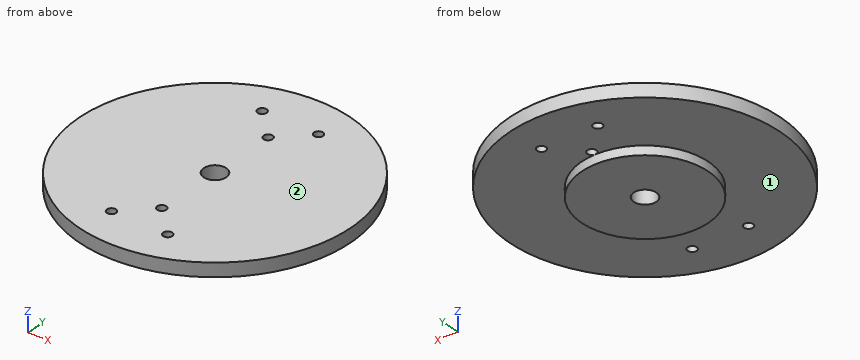
```python
from build123d import *

# Parameters (mm, degrees)
SKETCH1_R                = 76.2
SKETCH1_R_2              = 38.1
SKETCH1_R_3              = 12.7
SKETCH1_R_4              = 6.35
BOSS_EXTRUDE1_DEPTH      = 7.62
SKETCH2_R                = 35.56
BOSS_EXTRUDE2_DEPTH      = 5.08
CUT_EXTRUDE2_START       = -12.7
CUT_EXTRUDE2_OUTLINE_R   = 6.35
CUT_EXTRUDE2_OUTLINE_R_2 = 2.54
CUT_EXTRUDE2_DEPTH       = 12.7


# Read off the part's stored shape, not the designer's step: Cut-Extrude2
with BuildPart() as part:
    # Sketch1 → Boss-Extrude1 (new body)
    # profile 1 of 3: a face of its own
    with BuildSketch(Plane.XY):
        with Locations(Location((0, 0, 0), (0, 0, 180))):
            Circle(SKETCH1_R)
        Circle(SKETCH1_R_2, mode=Mode.SUBTRACT)
    # profile 2 of 3: a face of its own
    with BuildSketch(Plane.XY):
        Circle(SKETCH1_R_2)
        Circle(SKETCH1_R_3, mode=Mode.SUBTRACT)
    # profile 3 of 3: a face of its own
    with BuildSketch(Plane.XY):
        Circle(SKETCH1_R_3)
        with Locations(Location((0, 0, 0), (0, 0, 180))):
            Circle(SKETCH1_R_4, mode=Mode.SUBTRACT)
    extrude(amount=BOSS_EXTRUDE1_DEPTH)

    # Sketch2 → Boss-Extrude2 (add)
    with BuildSketch(Plane(origin=(0, 0, 0), x_dir=(-1, 0, 0), z_dir=(0, 0, -1))):
        with Locations(Location((0, 0, 0), (0, 0, 180))):
            Circle(SKETCH2_R)
    extrude(amount=BOSS_EXTRUDE2_DEPTH)

    # Cut-Extrude2 outline → Cut-Extrude2 (cut)
    with BuildSketch(Plane.XY.offset(7.62).offset(CUT_EXTRUDE2_START)):
        Circle(CUT_EXTRUDE2_OUTLINE_R)
        with Locations((-15.875, -53.975)):
            Circle(CUT_EXTRUDE2_OUTLINE_R_2)
        with Locations((0, -38.1)):
            Circle(CUT_EXTRUDE2_OUTLINE_R_2)
        with Locations((-15.875, 53.975)):
            Circle(CUT_EXTRUDE2_OUTLINE_R_2)
        with Locations((0, 38.1)):
            Circle(CUT_EXTRUDE2_OUTLINE_R_2)
        with Locations((15.875, 53.975)):
            Circle(CUT_EXTRUDE2_OUTLINE_R_2)
        with Locations((15.875, -53.975)):
            Circle(CUT_EXTRUDE2_OUTLINE_R_2)
    extrude(amount=CUT_EXTRUDE2_DEPTH, mode=Mode.SUBTRACT)


solid = part.part
```
CAD build for the part. Positions are in the model's coordinates, mm. Face numbers are marked on the shaded views. A direction names the side the tool comes from. Round coordinates to 2 decimals unless told otherwise and drop trailing zeros. Loops run counter-clockwise (first coordinate to the right, second up) from the corner with the lowest first, then second, coordinate; pieces in that order, holes last. Notation, with made-up numbers: M 71.5,-37.75 L 116.5,-37.75 A19 ccw 116.5,-33.75 Z; hole C 81,5.5 d10. An arc over 180 degrees is marked long. Use a Markdown table: item, result. Add a question column.
(1) Cut at A-A (y = 0). Give the cut face in (x, z).
(2) Cut at D-D (y = 38.1). Give the cut face in (x, z).
(3) Cut at B-B (x = -22.5). Give the cut face in (y, z), and give its area (3 significant figures).
(4) Drill centre lines: line 1 (Y direction, x = 0, z = 1.5); line 2 (Z direction, x = 56.5, y = 8.5); line 3 (X direction, y = 37.5, z = 0.5). Where is each one in solid material? Low to high.
(5) Which spindle directions (+Z, -Z, +X, -X, +Y, -Y) get a long thin tool onto all of the face, cutting with end or side? Do the marked faces 1 and 2. Say none if no direction does.
(6) Cut at C-C (z = -2.25). Give the cut face in (x, y), and give its area (3 significant figures).
(7) Flat gauge pins, fed straight in: pin 1 (3 mm diameter, centred on x = -22, y = -34, fed in from -Z); pin 2 (8 mm diameter, centred on x = 0, y = -38.1, fed in from +Z); pin 3 (2 mm diameter, centred on y = 10, z = -2, fed in from +X); pin 4 (1.5 mm diameter, centred on x = 9, z = 3, fed in from +Y). Where does each tip first touch, or does it go through?
Geometry says:
| question | item | result |
|---|---|---|
| 1 | outline | M -76.2,0 L -35.56,0 L -35.56,-5.08 L -6.35,-5.08 L -6.35,7.62 L -76.2,7.62 Z; M 6.35,-5.08 L 35.56,-5.08 L 35.56,0 L 76.2,0 L 76.2,7.62 L 6.35,7.62 Z |
| 2 | outline | M -65.99,0 L -2.54,0 L -2.54,7.62 L -65.99,7.62 Z; M 2.54,0 L 65.99,0 L 65.99,7.62 L 2.54,7.62 Z |
| 3 | outline | M -72.8,0 L -27.54,0 L -27.54,-5.08 L 27.54,-5.08 L 27.54,0 L 72.8,0 L 72.8,7.62 L -72.8,7.62 Z |
| 3 | area | 1,390 mm² |
| 4 | line 1 | y = -76.2 to -40.64, -35.56 to -6.35, 6.35 to 35.56, 40.64 to 76.2 |
| 4 | line 2 | z = 0 to 7.62 |
| 4 | line 3 | x = -66.33 to -2.47, 2.47 to 66.33 |
| 5 | face 1 | -Z |
| 5 | face 2 | +Z, +X, -X, +Y, -Y |
| 6 | outline | C 0,0 d71.12; hole C 0,0 d12.7 |
| 6 | area | 3,850 mm² |
| 7 | pin 1 | stops at z = 0 |
| 7 | pin 2 | stops at z = 7.62 |
| 7 | pin 3 | stops at x = 34.4 |
| 7 | pin 4 | stops at y = 75.75 |
